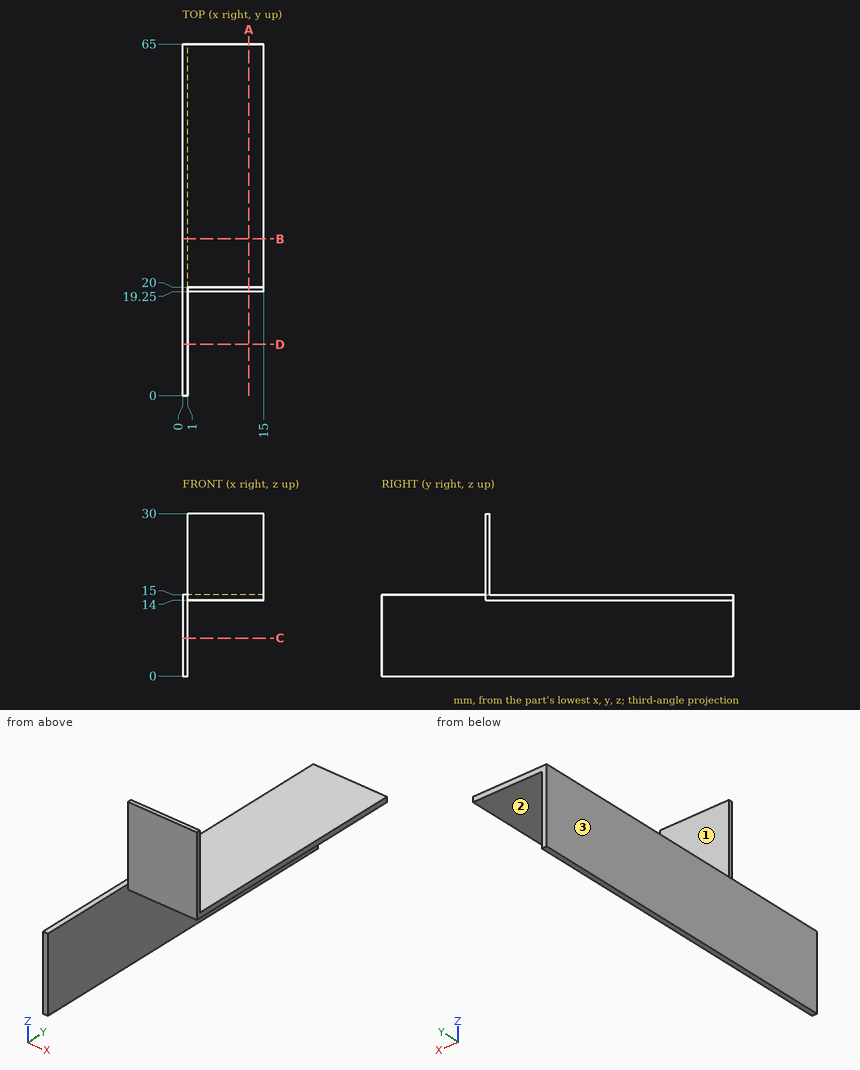
Could you check a few things on this drawing? It's one solid part, dimensions in mm from its lowest x, y, z. A direction names the side the tool comes from. Coordinates: 2 decimals unless noted, no trailing zeros. Order: outer loops, then holes, each group sorted by start corner. A loop starts at its lowest first (then second) coordinate and runs counter-clockwise, first axis right, second up. Notation, with made-up numbers: (-28, 24) - (-22, 24) arc R31 ccw to (-22, 57) - close; hole circle Ø10 at (50, -17). An arc over 180 degrees is marked (long way). Answer as a JSON object with one key per item and string values. Group by question number.
Q1. Will these pins go through, and if not, where does the flat tip stop? P1, Ø5, axis at x = 6, y = 24.5, coming from the +Z side; P2, Ø4, axis at x = 11.5, y = 52, coming from the -Z side; P3, Ø3, axis at y = 7.5, z = 12.5, coming from the +X side.
Q2. Imagine slicing it at B-B (y = 29). Please give me the cut outline in (x, z), and give its area (3 significant figures).
Q3. I need wall thicknesses on line 1 (Z direction, x = 13, y = 54); line 2 (Y direction, x = 3, z = 28.5); line 3 (X direction, y = 48.5, z = 11.75). Which ranges of each line are inside material? Lowest first, please. Write a range as from..to.
Q4. Imagine slicing it at D-D (y = 9.5). Please give me the cut outline in (x, z).
Q5. Imagine slicing it at C-C (z = 7). Please give me the cut outline in (x, y), and give its area (3 significant figures).
Q6. On a 3-axis mill with a long thin cutter (end or side, diameter ignored), from which of +Z, -Z, +X, -X, +Y, -Y can I reach the whole of each face in a straight line? I mean the marked faces 1, 2 and 3. Say none if no direction works.
Q7. Imagine slicing it at A-A (x = 12.25). Please give me the cut outline in (y, z), and give its area (3 significant figures).
Determined:
{
 "1": {"P1": "stops at z = 15", "P2": "stops at z = 14", "P3": "stops at x = 1"},
 "2": {"outline": "(0, 0) - (1, 0) - (1, 14) - (15, 14) - (15, 15) - (0, 15) - close", "area": "29.0 mm2"},
 "3": {"line 1": "z = 14..15", "line 2": "y = 19.25..20", "line 3": "x = 0..1"},
 "4": {"outline": "(0, 0) - (1, 0) - (1, 15) - (0, 15) - close"},
 "5": {"outline": "(0, 0) - (1, 0) - (1, 65) - (0, 65) - close", "area": "65.0 mm2"},
 "6": {"face 1": "+Z, +X, -X, +Y", "face 2": "-Z, +X, +Y, -Y", "face 3": "+Z, -Z, -X, +Y, -Y"},
 "7": {"outline": "(19.25, 14) - (65, 14) - (65, 15) - (20, 15) - (20, 30) - (19.25, 30) - close", "area": "57.0 mm2"}
}
